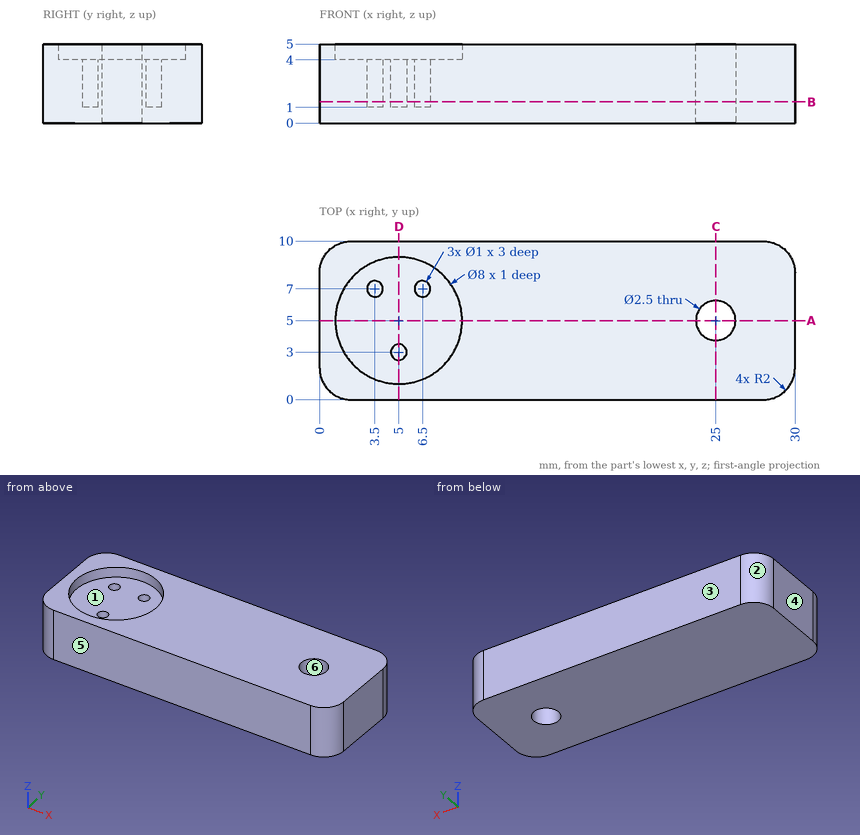
Can you work these out from the drawing? Everything is in mm from the part's minimum corner. A direction names the side the tool comes from. Give positions to 0.01 mm unless a question says otherwise; leave off trailing zeros. Order: outer loops, then holes, each group sorted by start corner. A loop starts at its lowest first (then second) coordinate and runs counter-clockwise, first axis right, second up. Notation, with made-up numbers: M 72.25,4.5 L 119.25,4.5 A11 cw 119.25,9.5 Z; hole C -14,7 d4. An arc over 180 degrees is marked long. Use a Markdown table: item, result. Add a question column.
1. For pin 1 Ø0.8 at (x, y) = (6.5, 7) entering from +Z; pin 2 Ø1.1 at (x, y) = (5, 3) entering from +Z, each with a flat end and sliding along its axis, tell me the tip position at first contact or that it passes through.
2. I need wall thicknesses on probe 1 along Y at (x, z) = (3.5, 2.05); probe 2 along Y at (x, z) = (5, 2.5); probe 3 along X at (y, z) = (5.75, 2.9). Which ranges of each line are inside material? Lowest first, please. Write a range as from..to.
3. If we mould it in two halves opening along Y, with no side actions, what happens to the marked faces 3, 4, 5 and 6? For each: +Y half, -Y half, draft (parallel to the pull), parting line (faces both ways), or undercut.
4. Suppose I cut it at D-D (x = 5). List the corners of the cut face in (y, z) for me.
5. Suppose I cut it at C-C (x = 25). List the corners of the cut face in (y, z) for me, and give its area (3 significant figures).
6. Suppose I cut it at A-A (y = 5). List the corners of the cut face in (x, z) for me, and give its area (4 significant figures).
7. On a 3-axis mill with a long thin cutter (end or side, diameter ignored), from which of +Z, -Z, +X, -X, +Y, -Y can I reach the whole of each face in a straight line? I mean the marked faces 1 and 2. Say none if no direction works.
8. Suppose I cut it at B-B (z = 1.35). List the corners of the cut face in (x, y) for me, and give its area (3 significant figures).
Results list:
| question | item | result |
|---|---|---|
| 1 | pin 1 | stops at z = 1 |
| 1 | pin 2 | stops at z = 4 |
| 2 | probe 1 | y = 0..6.5, 7.5..10 |
| 2 | probe 2 | y = 0..2.5, 3.5..10 |
| 2 | probe 3 | x = 0..24, 26..30 |
| 3 | face 3 | +Y half |
| 3 | face 4 | draft |
| 3 | face 5 | -Y half |
| 3 | face 6 | undercut |
| 4 | outline | M 0,0 L 10,0 L 10,5 L 9,5 L 9,4 L 3.5,4 L 3.5,1 L 2.5,1 L 2.5,4 L 1,4 L 1,5 L 0,5 Z |
| 5 | outline | M 0,0 L 3.75,0 L 3.75,5 L 0,5 Z; M 6.25,0 L 10,0 L 10,5 L 6.25,5 Z |
| 5 | area | 37.5 mm² |
| 6 | outline | M 0,0 L 23.75,0 L 23.75,5 L 9,5 L 9,4 L 1,4 L 1,5 L 0,5 Z; M 26.25,0 L 30,0 L 30,5 L 26.25,5 Z |
| 6 | area | 129.5 mm² |
| 7 | face 1 | +Z |
| 7 | face 2 | +Z, -Z, -X, +Y |
| 8 | outline | M 0,2 A2 ccw 2,0 L 28,0 A2 ccw 30,2 L 30,8 A2 ccw 28,10 L 2,10 A2 ccw 0,8 Z; hole C 3.5,7 d1; hole C 5,3 d1; hole C 6.5,7 d1; hole C 25,5 d2.5 |
| 8 | area | 289 mm² |
